Input: part model. Units: mm. Frame: model coordinates. A direction names the side the tool comes from. Coordinates: 2 decimals unless noted, no trailing zeros. Write each loop counter-clockwise with the first axis right and the second up, starting at its lowest first coordinate (ties: lowest second). Pieces come first, ordered by that corner, then holes. Notation, with made-up numbers: (-10, 72.25) - (-5, 72.25) arc R17 ccw to (-5, 94.25) - close; hole circle Ø2 at (42.5, -35.75). An arc over 180 degrees is marked (long way). Use a Markdown table: item, result. Add a question column.
Q1. Mould query, pull axis X, two halves, no side actions, for faces 5 (the face through (42.41, 7.986, 2.385)), 6 (the face through (-2.319, 7.986, -42.343)), 7 (the face through (-39.05, 5.03, -8.67)), 8 (the face through (-43, 9, 0)). Classes: released by +X, released by -X, zero draft, split by the parting line, or undercut.
Q2. Pin query (flat end, axial travel): P1, Ø5, axis at x = 1.5, z = 1, coming from the +Y side; P2, Ø1, axis at x = -1, z = 21.5, coming from the -Y side; P3, Ø8, axis at y = 1, z = -1.5, coming from the +X side; P4, Ø1, axis at y = -1.5, z = -7.5, coming from the +X side. Return the tip coordinate at first contact, or that it passes through.
Q3. Material intervals for probe 1 along X at (y, z) = (4.6, 0); probe 2 along Y at (x, z) = (-37, 8); probe 3 along X at (y, z) = (5, -31), sorted ascending. Write a range as from..to.
Q4. Section query A-A (z = 2). Return the cut outline in (x, y).
Q5. Set-up query: faces 1 (the face through (2.385, 7.986, -42.41)), 2 (the face through (-2.385, 7.986, 42.41)), 3 (the face through (-42.41, 7.986, -2.385)), 4 (the face through (-25.217, -3.944, -1.062)). Return all of +Z, -Z, +X, -X, +Y, -Y with unobstructed straight access to the full face (end or side cutting, diameter ignored); none if empty.
Q6. Section query C-C (z = -26). Return the cut outline in (x, y), then the cut area to 3 significant figures.
Q7. Section query B-B (x = 30). Return the cut outline in (y, z), then the cut area to 3 significant figures.
from build123d import *
from build123d.topology import SkipClean

# Parameters (mm, degrees)
SKETCH1_R           = 45
BOSS_EXTRUDE1_DEPTH = 7
SKETCH2_R           = 40
CUT_EXTRUDE1_DEPTH  = 4
SKETCH3_R           = 5
BOSS_EXTRUDE2_DEPTH = 4
BOSS_EXTRUDE3_DEPTH = 2
CIRPATTERN1_COUNT   = 4
SKETCH5_R           = 4.9
BOSS_EXTRUDE4_DEPTH = 8


with BuildPart() as part:
    # Sketch1 → Boss-Extrude1 (new body)
    with BuildSketch(Plane(origin=(0, 0, 0), x_dir=(1, 0, 0), z_dir=(0, 1, 0))):
        with Locations(Location((0, 0, 0), (0, 0, 270))):
            Circle(SKETCH1_R)
    extrude(amount=BOSS_EXTRUDE1_DEPTH)

    # Sketch2 → Cut-Extrude1 (cut)
    with BuildSketch(Plane(origin=(0, 7, 0), x_dir=(1, 0, 0), z_dir=(0, 1, 0))):
        with Locations(Location((0, 0, 0), (0, 0, 270))):
            Circle(SKETCH2_R)
    extrude(amount=-CUT_EXTRUDE1_DEPTH, mode=Mode.SUBTRACT)

    # Sketch3 → Boss-Extrude2 (add)
    with BuildSketch(Plane(origin=(0, 3, 0), x_dir=(1, 0, 0), z_dir=(0, 1, 0))):
        with Locations(Location((0, 0, 0), (0, 0, 270))):
            Circle(SKETCH3_R)
    extrude(amount=BOSS_EXTRUDE2_DEPTH)

    # Sketch4 → Boss-Extrude3 (add)
    with SkipClean():  # the faces are left unmerged after this step: merging them gives an invalid solid
        with BuildSketch(Plane(origin=(0, 7, 0), x_dir=(1, 0, 0), z_dir=(0, 1, 0))):
            with BuildLine():
                Line((0, 40), (-4.703780847, 44.753485292))
                ThreePointArc((-4.703780847, 44.753485292), (0, 45), (4.703780847, 44.753485292))
                Line((4.703780847, 44.753485292), (0, 40))
            make_face()
        boss_extrude3 = extrude(amount=BOSS_EXTRUDE3_DEPTH)

    # CirPattern1: Boss-Extrude3 ×4 about axis
    with SkipClean():  # the faces are left unmerged after this step: merging them gives an invalid solid
        cirpattern1_axis = Axis((0, 0, 0), (0, 1, 0))
        for i in range(1, CIRPATTERN1_COUNT):
            add(boss_extrude3.rotate(cirpattern1_axis, i * 360 / CIRPATTERN1_COUNT))

    # Sketch5 → Boss-Extrude4 (add)
    with SkipClean():  # the faces are left unmerged after this step: merging them gives an invalid solid
        with BuildSketch(Plane(origin=(0, 0, 0), x_dir=(-1, 0, 0), z_dir=(0, -1, 0))):
            with Locations(Location((30, 0, 0), (0, 0, 270))):
                Circle(SKETCH5_R)
        boss_extrude4 = extrude(amount=BOSS_EXTRUDE4_DEPTH)

    # Mirror1: Boss-Extrude4 across plane
    with SkipClean():  # the faces are left unmerged after this step: merging them gives an invalid solid
        add(boss_extrude4.mirror(Plane(origin=(0, 0, 0), x_dir=(0, 0, 1), z_dir=(1, 0, 0))))


solid = part.part
Values follow:
| question | item | result |
|---|---|---|
| 1 | face 5 | undercut |
| 1 | face 6 | released by -X |
| 1 | face 7 | undercut |
| 1 | face 8 | zero draft |
| 2 | P1 | y = 7 |
| 2 | P2 | y = 0 |
| 2 | P3 | x = 45 |
| 2 | P4 | through |
| 3 | probe 1 | -45..-40, -5..5, 40..45 |
| 3 | probe 2 | 0..3 |
| 3 | probe 3 | -32.62..-25.28, 25.28..32.62 |
| 4 | outline | (-44.96, 0) - (-34.47, 0) - (-34.47, -8) - (-25.53, -8) - (-25.53, 0) - (25.53, 0) - (25.53, -8) - (34.47, -8) - (34.47, 0) - (44.96, 0) - (44.96, 9) - (42.02, 9) - (42.02, 7) - (39.95, 7) - (39.95, 3) - (4.58, 3) - (4.58, 7) - (-4.58, 7) - (-4.58, 3) - (-39.95, 3) - (-39.95, 7) - (-42.02, 7) - (-42.02, 9) - (-44.96, 9) - close |
| 5 | face 1 | +X, +Y |
| 5 | face 2 | -X, +Y |
| 5 | face 3 | -Z, +Y |
| 5 | face 4 | -Y |
| 6 | outline | (-36.73, 0) - (36.73, 0) - (36.73, 7) - (30.4, 7) - (30.4, 3) - (-30.4, 3) - (-30.4, 7) - (-36.73, 7) - close |
| 6 | area | 271 mm2 |
| 7 | outline | (-8, -4.9) - (0, -4.9) - (0, -33.54) - (7, -33.54) - (7, -26.46) - (3, -26.46) - (3, 26.46) - (7, 26.46) - (7, 33.54) - (0, 33.54) - (0, 4.9) - (-8, 4.9) - close |
| 7 | area | 336 mm2 |
